The model under review builds one solid part; all positions refer to its coordinate system, in mm. A direction names the side the tool comes from. Round coordinates to 2 decimals unless told otherwise and drop trailing zeros. Loops run counter-clockwise (first coordinate to the right, second up) from the corner with the lowest first, then second, coordinate; pieces in that order, holes last. Notation, with made-up numbers: M 70,-5.75 L 109,-5.75 A18 cw 109,15.25 Z; hole C 1.5,-39 d10. An arc over 180 degrees is marked long. Answer as a JSON object with one key per item and string values. Group by question number.
Item 1: To check wall thickness, follow line 1 (Y direction, x = 240, z = 96); line 2 (Z direction, x = 177.5, y = 2.5); line 3 (Z direction, x = 30, y = 29). State the ranges of each line that lie inside material, in increasing order.
Item 2: Insertion check: P1, Ø1.5, axis at y = -2.5, z = -75, coming from the +X side; P2, Ø4, axis at x = 105.5, y = 1, coming from the +Z side; P3, Ø12.5, axis at x = 60, z = 146.5, coming from the +Y side. Each pin has a flat end and moves straight along its axis. Give the tip position at first contact, or say it passes through.
Item 3: Consider section A-A (x = 126). Give the boundary of the cut face in (y, z).
Item 4: Consider section C-C (x = 60). Give the boundary of the cut face in (y, z), and give its area (3 significant figures).
Item 5: Tool access review of faces 5 (the face through (0, 0, -2)), 6 (the face through (61.627, 28.07, 162.394)), 7 (the face through (232, 8, 27)): name each direction out of +Z, -Z, +X, -X, +Y, -Y from which nothing blocks a thin tool from reaching the whole face with its end or side.
Item 6: Consider section B-B (z = 22.5). Give the boundary of the cut face in (x, y), and give its area (3 significant figures).
Item 7: The part is to be moulded in two halves that separate along X. For faces 1 (the face through (60, 23, 150)), 2 (the face through (250, 20, -2)), 3 (the face through (232, -8, -27)), 4 (the face through (31.627, 28.07, 162.394)), say which applies: +X half, -X half, draft (parallel to the pull), parting line (faces both ways), or undercut.
```python
from build123d import *

# Parameters (mm, degrees)
F3_R     = 12.5
F4_DEPTH = 10
F6_DEPTH = 30
F7_R     = 5


with BuildPart() as f2:
    # F2: sweep along a path in F1
    with BuildLine(Plane.XZ) as f2_path:
        Line((0, 0), (250, 0))
    # F0 (on Right) → F2 (sweep)
    with BuildSketch(Plane.YZ):
        Polygon((8, 150), (0, 150), (-8, 150), (-8, 180), (-33, 180), (-33, -180), (-8, -180), (-8, -150), (0, -150), (8, -150), (8, -180), (33, -180), (33, 180), (8, 180), align=None)
    sweep(path=f2_path.line)

    # F3 (on face) → F4 (cut)
    with BuildSketch(Plane(origin=(0, 33, 0), x_dir=(-1, 0, 0), z_dir=(0, 1, 0))):
        with Locations((-60, 150)):
            Circle(F3_R)
        with Locations((-30, 150)):
            Circle(F3_R)
    extrude(amount=-F4_DEPTH, mode=Mode.SUBTRACT)

    # F5 (on face) → F6 (cut)
    with BuildSketch(Plane.YZ.offset(250)):
        Polygon((8, 150), (0, 150), (-8, 150), (-8, -150), (0, -150), (8, -150), align=None)
    extrude(amount=-F6_DEPTH, mode=Mode.SUBTRACT)

    # F7
    f7_edges = [f2.edges().sort_by_distance(p)[0] for p in [
        (110, 8, 150),
        (220, 0, 150),
        (110, -8, 150),
        (0, 0, 150),
        (110, -8, -150),
        (220, 0, -150),
        (110, 8, -150),
        (0, 0, -150),
        (125, 8, -180),
        (0, 20.5, -180),
        (125, 33, -180),
        (250, 20.5, -180),
        (125, 33, 180),
        (0, 20.5, 180),
        (125, 8, 180),
        (250, 20.5, 180),
        (125, -8, 180),
        (0, -20.5, 180),
        (125, -33, 180),
        (250, -20.5, 180),
        (125, -33, -180),
        (0, -20.5, -180),
        (125, -8, -180),
        (250, -20.5, -180),
        (0, -8, 165),
        (0, -8, -165),
        (0, 8, -165),
        (0, 8, 165),
        (250, 8, 0),
        (250, 33, 0),
        (250, -8, 0),
        (250, -33, 0),
        (220, -8, 0),
        (220, 8, 0),
    ]]
    fillet(f7_edges, radius=F7_R)


solid = f2.part
```
Geometry results:
{
 "1": {"line 1": "y = -33 to -8, 8 to 33", "line 2": "z = -150 to 150", "line 3": "z = -179.9 to 137.5, 162.5 to 179.9"},
 "2": {"P1": "stops at x = 220.01", "P2": "stops at z = 150", "P3": "stops at y = 23"},
 "3": {"outline": "M -33,-175 A5 ccw -28,-180 L -13,-180 A5 ccw -8,-175 L -8,-155 A5 cw -3,-150 L 3,-150 A5 cw 8,-155 L 8,-175 A5 ccw 13,-180 L 28,-180 A5 ccw 33,-175 L 33,175 A5 ccw 28,180 L 13,180 A5 ccw 8,175 L 8,155 A5 cw 3,150 L -3,150 A5 cw -8,155 L -8,175 A5 ccw -13,180 L -28,180 A5 ccw -33,175 Z"},
 "4": {"outline": "M -33,-175 A5 ccw -28,-180 L -13,-180 A5 ccw -8,-175 L -8,-155 A5 cw -3,-150 L 3,-150 A5 cw 8,-155 L 8,-175 A5 ccw 13,-180 L 28,-180 A5 ccw 33,-175 L 33,137.5 L 23,137.5 L 23,162.5 L 33,162.5 L 33,175 A5 ccw 28,180 L 13,180 A5 ccw 8,175 L 8,155 A5 cw 3,150 L -3,150 A5 cw -8,155 L -8,175 A5 ccw -13,180 L -28,180 A5 ccw -33,175 Z", "area": "22,500 mm^2"},
 "5": {"face 5": "+Z, -Z, -X, +Y, -Y", "face 6": "+Y", "face 7": "+X"},
 "6": {"outline": "M 0,-33 L 245,-33 A5 ccw 250,-28 L 250,-13 A5 ccw 245,-8 L 225,-8 A5 cw 220,-3 L 220,3 A5 cw 225,8 L 245,8 A5 ccw 250,13 L 250,28 A5 ccw 245,33 L 0,33 Z", "area": "16,000 mm^2"},
 "7": {"face 1": "undercut", "face 2": "+X half", "face 3": "draft", "face 4": "undercut"}
}
